```python
from build123d import *

# Parameters (mm, degrees)
F1_DEPTH = 1.5875
F4_W     = 19.05
F4_H     = 1.5875
F5_DEPTH = 1.5875


with BuildPart() as f1:
    # F0 (on Front) → F1 (new body)
    with BuildSketch(Plane.XZ):
        with BuildLine():
            ThreePointArc((4.4277010242, -1.7541008779), (4.6780515377, -0.8928830052), (4.7625, 0))
            ThreePointArc((4.7625, 0), (-0.8928830052, 4.6780515377), (-4.4277010242, -1.7541008779))
            ThreePointArc((-4.4277010242, -1.7541008779), (0, -4.7625), (4.4277010242, -1.7541008779))
        make_face()
        with BuildLine():
            ThreePointArc((-4.4277010242, -1.7541008779), (-0.8928830052, 4.6780515377), (4.7625, 0))
            ThreePointArc((4.7625, 0), (4.6780515377, -0.8928830052), (4.4277010242, -1.7541008779))
            Line((4.4277010242, -1.7541008779), (9.525, 11.1125))
            Line((9.525, 11.1125), (-9.525, 11.1125))
            Line((-9.525, 11.1125), (-4.4277010242, -1.7541008779))
        make_face()
    extrude(amount=F1_DEPTH)

    # F2 (on Top) → F3 (revolve)
    with BuildSketch(Plane.XY):
        with BuildLine():
            Line((0, 0), (3.175, 0))
            Line((3.175, 0), (3.175, 7.5627420857))
            ThreePointArc((3.175, 7.5627420857), (1.6993652025, 6.6635041404), (0, 6.35))
            Line((0, 6.35), (0, 0))
        make_face()
        with BuildLine():
            ThreePointArc((0, 6.35), (1.6993652025, 6.6635041404), (3.175, 7.5627420857))
            ThreePointArc((3.175, 7.5627420857), (4.4489958596, 12.8118652025), (0, 15.875))
            Line((0, 15.875), (0, 11.1125))
            Line((0, 11.1125), (0, 6.35))
        make_face()
    revolve(axis=Axis((0, 5.55625, 0), (0, -1, 0)))

    # F4 (on face) → F5 (join)
    with BuildSketch(Plane.XY.offset(11.1125)):
        with BuildLine():
            Line((9.525, -1.5875), (15.08125, -1.5875))
            ThreePointArc((15.08125, -1.5875), (22.225, 5.55625), (15.08125, 12.7))
            Line((15.08125, 12.7), (-15.08125, 12.7))
            ThreePointArc((-15.08125, 12.7), (-22.225, 5.55625), (-15.08125, -1.5875))
            Line((-15.08125, -1.5875), (-9.525, -1.5875))
            Line((-9.525, -1.5875), (-9.525, 0))
            Line((-9.525, 0), (9.525, 0))
            Line((9.525, 0), (9.525, -1.5875))
        make_face()
        with BuildLine():
            ThreePointArc((-17.065625, 3.571875), (-19.05, 5.55625), (-17.065625, 7.540625))
            Line((-17.065625, 7.540625), (-6.746875, 7.540625))
            ThreePointArc((-6.746875, 7.540625), (-4.7625, 5.55625), (-6.746875, 3.571875))
            Line((-6.746875, 3.571875), (-17.065625, 3.571875))
        make_face(mode=Mode.SUBTRACT)
        with BuildLine():
            ThreePointArc((17.065625, 7.540625), (19.05, 5.55625), (17.065625, 3.571875))
            Line((17.065625, 3.571875), (6.746875, 3.571875))
            ThreePointArc((6.746875, 3.571875), (4.7625, 5.55625), (6.746875, 7.540625))
            Line((6.746875, 7.540625), (17.065625, 7.540625))
        make_face(mode=Mode.SUBTRACT)
        with Locations((0, -0.79375)):
            Rectangle(F4_W, F4_H)
    extrude(amount=F5_DEPTH)


solid = f1.part
```
Read the model definition and answer for the solid it produces. Units are mm, in the model's axes. A direction names the side the tool comes from. Give positions to 0.01 mm unless a question says otherwise; leave off trailing zeros. Write each loop counter-clockwise with the first axis right and the second up, starting at its lowest first coordinate (ties: lowest second). Pieces come first, ordered by that corner, then holes. Notation, with made-up numbers: (41.5, -12.75) -> (71.5, -12.75) arc R16 ccw to (71.5, -8.75) -> close; hole circle Ø9 at (62, -6). An arc over 180 degrees is marked (long way). Answer in a Markdown table with one row per item.
1) Section A-A on x = -11.5 is taken. Give the vertices of the cut face in (y, z).
Results list:
| item | result |
|---|---|
| outline | (-1.59, 11.11) -> (3.57, 11.11) -> (3.57, 12.7) -> (-1.59, 12.7) -> close; (7.54, 11.11) -> (12.7, 11.11) -> (12.7, 12.7) -> (7.54, 12.7) -> close |
2) Determine the mould class of faces 3 (the cylindrical face through (-0.69, 3.83, -3.1)), 4 (the flat face through (6.94, -0.78, 4.59)), 5 (the flat face through (0, 12.7, 12)) for opening direction Y: released by +Y, released by -Y, zero draft, split by the parting line, or undercut.
Results list:
| item | result |
|---|---|
| face 3 | undercut |
| face 4 | zero draft |
| face 5 | released by +Y |
3) Straight lines are drawn through the part: line 1 (X direction, y = 7, z = 12); line 2 (Z direction, x = 13, y = 0); line 3 (Y direction, x = 3, z = 1.25). For each, find the intervals that lie inside material, in ascending order. Write a range as [from, to].
Results list:
| item | result |
|---|---|
| line 1 | [-22.08, -18.43], [-5.39, 5.39], [18.43, 22.08] |
| line 2 | [11.11, 12.7] |
| line 3 | [-1.59, 0], [7.63, 14.59] |
4) Each of these flat-tipped pins is pushed along its axis until it touches: pin 1 Ø5 at (y, z) = (12.5, -1.5) entering from -X; pin 2 Ø4.5 at (x, y) = (4.5, 4) entering from -Z; pin 3 Ø0.8 at (x, z) = (-10, 11.5) entering from +Y. Where does it stop, or does it pass through?
Results list:
| item | result |
|---|---|
| pin 1 | x = -4.76 |
| pin 2 | z = -2.24 |
| pin 3 | y = 12.7 |
5) Section B-B on y = 6.5 is taken. Count the separate pieces of the cut face and the enclosed holes in it, plus the area to 3 significant figures.
Results list:
| item | result |
|---|---|
| separate pieces | 4 |
| enclosed holes | 0 |
| area | 58.2 mm^2 |
6) Section D-D on z = 2.25 is taken. Give the vertices of the cut face in (x, y).
Results list:
| item | result |
|---|---|
| outline | (-6.01, -1.59) -> (6.01, -1.59) -> (6.01, 0) -> (2.24, 0) -> (2.24, 7.56) arc R4.2 ccw (long way) to (-2.24, 7.56) -> (-2.24, 0) -> (-6.01, 0) -> close |
7) A tool of negligible diameter and unlimited length cuts with its end or side. For faces 1 (the cylindrical face through (-22.223, 5.713, 11.895)), 2 (the cylindrical face through (-4.763, 5.6, 11.895)), from which of +Z, -Z, +X, -X, +Y, -Y can it reach the whole face along a straight path? Write none if from no direction.
Results list:
| item | result |
|---|---|
| face 1 | +Z, -Z, -X |
| face 2 | +Z, -Z |
8) Section C-C on x = 0 is taken. Give the vertices of the cut face in (y, z) (1 decimal), plus the area to 3 significant figures.
Results list:
| item | result |
|---|---|
| outline | (-1.6, -4.8) -> (0, -4.8) -> (0, -3.2) -> (7.6, -3.2) arc R4.8 ccw (long way) to (7.6, 3.2) -> (0, 3.2) -> (0, 11.1) -> (12.7, 11.1) -> (12.7, 12.7) -> (-1.6, 12.7) -> close |
| area | 162 mm^2 |
